Geometry check sheet. Reference: the model listing, model coordinates, mm. Face numbers are marked on the shaded views. A direction names the side the tool comes from. Round coordinates to 2 decimals unless told otherwise and drop trailing zeros. Write each loop counter-clockwise with the first axis right and the second up, starting at its lowest first coordinate (ties: lowest second). Pieces come first, ordered by that corner, then holes. Notation, with made-up numbers: M -20,86 L 18,86 A13 cw 18,94 Z; hole C 81.5,68 d6. An arc over 180 degrees is marked long. One line per item, written item: value. Start each with the question number.
1. Scan lines: probe 1 along Y at (x, z) = (55.5, 152.4); probe 2 along Z at (x, y) = (4, -2) (3 decimals); probe 3 along Y at (x, z) = (35, 304.8). Record each from-to range of solid material in increasing order. Write a range as [from, to].
2. Section check C-C (z = 72.5). Record the boundary of the cut face in (x, y), and give its area (3 significant figures).
3. Access from +Z, -Z, +X, -X, +Y, -Y to the whole of each face (thin tool, end or side, straight path). Record for the marked faces 1, 2 and 3.
4. Depth check by flat-ended pin: P1, Ø11.5, axis at y = 0, z = 58, coming from the +X side; P2, Ø3, axis at y = -5.5, z = 168, coming from the -X side; P3, Ø19, axis at x = 59.5, y = 0.5, coming from the +Z side; P4, Ø8, axis at x = 27, y = 7.5, coming from the +Z side. Enter the tip coordinate at first touch or a pass-through.
5. Section check A-A (z = 152.4). Record the boundary of the cut face in (x, y), and give its area (3 significant figures).
from build123d import *

# Parameters (mm, degrees)
SKETCH1_R           = 14.2875
BOSS_EXTRUDE1_DEPTH = 38.1
SKETCH2_W           = 76.2
SKETCH2_H           = 38.1
SKETCH2_R           = 14.2875
BOSS_EXTRUDE2_DEPTH = 38.1
CUT_EXTRUDE1_DEPTH  = 38.1
FILLET1_R           = 12.7
SKETCH4_W           = 38.1
SKETCH4_H           = 38.1
BOSS_EXTRUDE3_DEPTH = 152.4
SKETCH5_R           = 4
CUT_EXTRUDE2_DEPTH  = 152.4
SKETCH6_W           = 25
SKETCH6_H           = 54.519891076
CUT_EXTRUDE3_DEPTH  = 152.4


with BuildPart() as part:
    # Sketch1 → Boss-Extrude1 (new body)
    with BuildSketch(Plane(origin=(0, 0, 0), x_dir=(0, 0, -1), z_dir=(1, 0, 0))):
        with BuildLine():
            Line((29.337186502, -19.05), (-175.255687154, -19.05))
            Line((-175.255687154, -19.05), (-175.255687154, 19.05))
            Line((-175.255687154, 19.05), (29.337186502, 19.05))
            Line((29.337186502, 19.05), (29.337186502, 4))
            Line((29.337186502, 4), (13.442493258, 4))
            ThreePointArc((13.442493258, 4), (0, 14.025), (-13.442493258, 4))
            Line((-13.442493258, 4), (-18.025, 4))
            Line((-18.025, 4), (-18.025, -4))
            Line((-18.025, -4), (-13.442493258, -4))
            ThreePointArc((-13.442493258, -4), (0, -14.025), (13.442493258, -4))
            Line((13.442493258, -4), (29.337186502, -4))
            Line((29.337186502, -4), (29.337186502, -19.05))
        make_face()
        with Locations(Location((-152.4, 0, 0), (0, 0, 180))):
            Circle(SKETCH1_R, mode=Mode.SUBTRACT)
    extrude(amount=BOSS_EXTRUDE1_DEPTH)

    # Sketch2 → Boss-Extrude2 (add)
    with BuildSketch(Plane(origin=(38.1, 0, 0), x_dir=(0, 0, -1), z_dir=(1, 0, 0))):
        with Locations((-137.155687154, 0)):
            Rectangle(SKETCH2_W, SKETCH2_H)
        with Locations(Location((-152.4, 0, 0), (0, 0, 180))):
            Circle(SKETCH2_R, mode=Mode.SUBTRACT)
    extrude(amount=BOSS_EXTRUDE2_DEPTH)

    # Sketch3 → Cut-Extrude1 (cut)
    with BuildSketch(Plane(origin=(0, 19.05, 0), x_dir=(1, 0, 0), z_dir=(0, 1, 0))):
        Polygon((38.1, -99.055687154), (76.2, -132.562404594), (94.277321555, -84.449227978), align=None)
    extrude(amount=-CUT_EXTRUDE1_DEPTH, mode=Mode.SUBTRACT)

    # Fillet1
    fillet1_edges = [part.edges().sort_by_distance(p)[0] for p in [
        (38.1, 0, 99.055687154),
    ]]
    fillet(fillet1_edges, radius=FILLET1_R)

    # Sketch4 → Boss-Extrude3 (add)
    with BuildSketch(Plane.XY.offset(175.255687154)):
        with Locations((19.05, 0)):
            Rectangle(SKETCH4_W, SKETCH4_H)
    extrude(amount=BOSS_EXTRUDE3_DEPTH)

    # Sketch5 → Cut-Extrude2 (cut)
    with BuildSketch(Plane.ZY):
        Polygon((276.061983206, 26.741787919), (276.061983206, 19.05), (327.655687154, 19.05), (327.655687154, -19.05), (276.061983206, -19.05), (276.061983206, -31.426856949), (335.038222157, -31.426856949), (335.038222157, 26.741787919), align=None)
        with BuildLine():
            Line((327.655687154, 19.05), (276.061983206, 19.05))
            ThreePointArc((276.061983206, 19.05), (281.943389767, 18.165675684), (287.304689246, 15.590905686))
            ThreePointArc((287.304689246, 15.590905686), (295.144592117, 12.051491747), (303.720086759, 11.378870216))
            ThreePointArc((303.720086759, 11.378870216), (312.490952205, 8.455421585), (316.23, 0))
            ThreePointArc((316.23, 0), (312.381148337, -8.554010165), (303.426659685, -11.347195089))
            ThreePointArc((303.426659685, -11.347195089), (296.515249828, -11.473357637), (289.902590337, -13.487367982))
            ThreePointArc((289.902590337, -13.487367982), (283.520288655, -17.607307989), (276.061983206, -19.05))
            Line((276.061983206, -19.05), (327.655687154, -19.05))
            Line((327.655687154, -19.05), (327.655687154, 19.05))
        make_face()
        with Locations((304.8, 0)):
            Circle(SKETCH5_R)
    extrude(amount=-CUT_EXTRUDE2_DEPTH, mode=Mode.SUBTRACT)

    # Sketch6 → Cut-Extrude3 (cut)
    with BuildSketch(Plane.XZ.offset(19.05)):
        with Locations((19.05, 316.23)):
            Rectangle(SKETCH6_W, SKETCH6_H)
    extrude(amount=-CUT_EXTRUDE3_DEPTH, mode=Mode.SUBTRACT)


solid = part.part
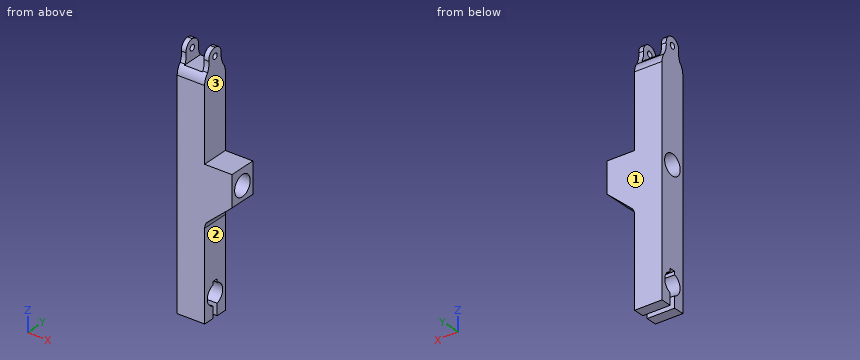
Result sheet:
1. probe 1: y = [-19.05, -14.29], [14.29, 19.05]
1. probe 2: z = [18.025, 138.253], [166.547, 301.336], [308.264, 316.054]
1. probe 3: y = [-11.43, -4], [4, 11.43]
2. outline: M 0,-19.05 L 38.1,-19.05 L 38.1,19.05 L 0,19.05 Z
2. area: 1,450 mm2
3. face 1: +Z, -Z, +X, -X, +Y
3. face 2: -Z, +X, +Y, -Y
3. face 3: +Z, +X, +Y, -Y
4. P1: stops at x = 38.1
4. P2: stops at x = 0
4. P3: stops at z = 175.26
4. P4: stops at z = 288.97
5. outline: M 0,-19.05 L 76.2,-19.05 L 76.2,-14.29 L 0,-14.29 Z; M 0,14.29 L 76.2,14.29 L 76.2,19.05 L 0,19.05 Z
5. area: 726 mm2
